Check sheet for the drawn part. Datum: minimum x, y, z corner. Units: mm. A direction names the side the tool comes from. Round coordinates to 2 decimals unless told otherwise and drop trailing zeros. Order: outer loops, then holes, each group sorted by start corner. A loop starts at its lowest first (then second) coordinate and runs counter-clockwise, first axis right, second up.
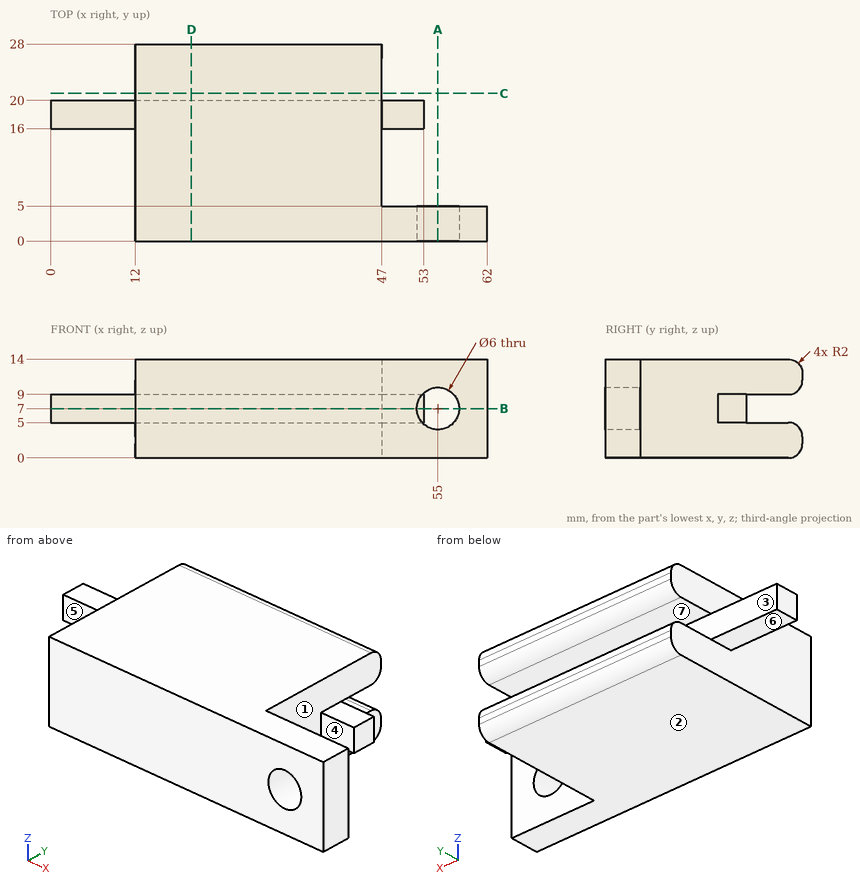
(1) Depth check by flat-ended pin: P1, Ø4.5, axis at x = 6, y = 18, coming from the +Z side; P2, Ø7, axis at y = 14.5, z = 6.5, coming from the +X side; P3, Ø7, axis at x = 52.5, z = 9, coming from the +Y side. Enter the tip coordinate at first touch or a pass-through.
Returned:
P1: stops at z = 9
P2: stops at x = 53
P3: stops at y = 20
(2) Sectioned sample at B-B, the plane z = 7. Record the cut outline in (x, y), and give its area (3 significant figures).
Returned:
outline: (0, 16) - (12, 16) - (12, 0) - (52, 0) - (52, 5) - (47, 5) - (47, 16) - (53, 16) - (53, 20) - (0, 20) - close; (58, 0) - (62, 0) - (62, 5) - (58, 5) - close
area: 817 mm2
(3) Set-up check for the marked faces 4, 5, 6 and 7: record each of +Z, -Z, +X, -X, +Y, -Y from which the full face is reachable in a straight line by a thin tool's end or side.
Returned:
face 4: +Z, -Z, +X
face 5: +Z, -Z, -X, -Y
face 6: -Z, -X, +Y, -Y
face 7: +X, -X, +Y
(4) Sectioned sample at A-A, the plane x = 55. Record the cut outline in (y, z).
Returned:
outline: (0, 0) - (5, 0) - (5, 4) - (0, 4) - close; (0, 10) - (5, 10) - (5, 14) - (0, 14) - close
(5) Sectioned sample at D-D, the plane x = 20. Record the cut outline in (y, z), and give its area (3 significant figures).
Returned:
outline: (0, 0) - (26, 0) arc R2 ccw to (28, 2) - (28, 3) arc R2 ccw to (26, 5) - (20, 5) - (20, 9) - (26, 9) arc R2 ccw to (28, 11) - (28, 12) arc R2 ccw to (26, 14) - (0, 14) - close
area: 357 mm2
(6) Material ranges on line 1 (Z direction, x = 39, y = 24.25); line 2 (X direction, y = 1.75, z = 7); line 3 (X direction, y = 16.75, z = 2), recorded low to high.
Returned:
line 1: z = 0 to 5, 9 to 14
line 2: x = 12 to 52, 58 to 62
line 3: x = 12 to 47
(7) Draft check along Y on the marked faces 1, 2 and 3. Enter one of: released by +Y, released by -Y, zero draft, split by the parting line, or undercut.
Returned:
face 1: undercut
face 2: zero draft
face 3: released by +Y
(8) Sectioned sample at C-C, the plane y = 21. Record the cut outline in (x, z), and give its area (3 significant figures).
Returned:
outline: (12, 0) - (47, 0) - (47, 5) - (12, 5) - close; (12, 9) - (47, 9) - (47, 14) - (12, 14) - close
area: 350 mm2
